```python
from build123d import *

# Parameters (mm, degrees)
SKETCH_1_W        = 29
SKETCH_1_H        = 15
SKETCH_1_R        = 1.5
SKETCH_1_R_2      = 2.5
EXTRUDE_1_DEPTH   = 3
SKETCH_1_3_R      = 4
SKETCH_1_3_R_2    = 2.5
EXTRUDE_1_2_DEPTH = 15
FILLET_1_R        = 2


with BuildPart() as part:
    # 草图1 → Extrude 1 (new body)
    # profile 1 of 2: a face of its own
    with BuildSketch(Plane.XY):
        with Locations((14.5, 7.5)):
            Rectangle(SKETCH_1_W, SKETCH_1_H)
        with Locations((9.5, 2.5)):
            Circle(SKETCH_1_R, mode=Mode.SUBTRACT)
        with Locations((9.5, 12.5)):
            Circle(SKETCH_1_R, mode=Mode.SUBTRACT)
        with Locations((26.5, 7.5)):
            Circle(SKETCH_1_R, mode=Mode.SUBTRACT)
        with Locations((2.5, 7.5)):
            Circle(SKETCH_1_R, mode=Mode.SUBTRACT)
        with Locations((14.5, 7.5)):
            Circle(SKETCH_1_R_2, mode=Mode.SUBTRACT)
    # profile 2 of 2: a face of its own
    with BuildSketch(Plane.XY):
        with Locations((14.5, 7.5)):
            Circle(SKETCH_1_R_2)
    extrude(amount=EXTRUDE_1_DEPTH)

    # 草图1<3> → Extrude 1 2 (add)
    with BuildSketch(Plane.XY):
        with Locations((14.5, 7.5)):
            Circle(SKETCH_1_3_R)
        with Locations((14.5, 7.5)):
            Circle(SKETCH_1_3_R_2, mode=Mode.SUBTRACT)
    extrude(amount=EXTRUDE_1_2_DEPTH)

    # 圆角1
    fillet_1_edges = [part.edges().sort_by_distance(p)[0] for p in [
        (0, 0, 1.5),
        (0, 15, 1.5),
        (29, 15, 1.5),
        (29, 0, 1.5),
    ]]
    fillet(fillet_1_edges, radius=FILLET_1_R)


solid = part.part
```
The listing builds one solid part. Answer for the finished solid, in the listing's coordinates (mm). A direction names the side the tool comes from. Coordinates: 2 decimals unless noted, no trailing zeros. Write each loop counter-clockwise with the first axis right and the second up, starting at its lowest first coordinate (ties: lowest second). Pieces come first, ordered by that corner, then holes.
Q1. Section B-B, the plane y = 7.5 is taken. Write down the section's boundary in (x, z), then the cut area to 3 significant figures.
Returned:
outline: (0, 0) - (1, 0) - (1, 3) - (0, 3) - close; (4, 0) - (25, 0) - (25, 3) - (18.5, 3) - (18.5, 15) - (17, 15) - (17, 3) - (12, 3) - (12, 15) - (10.5, 15) - (10.5, 3) - (4, 3) - close; (28, 0) - (29, 0) - (29, 3) - (28, 3) - close
area: 105 mm2
Q2. Find the intervals of material crossed by line 1 along X through (y, z) = (7.5, 14); line 2 along Y through (x, z) = (14.5, 9.75); line 3 along Y through (x, z) = (26.5, 1.3), in increasing order.
Returned:
line 1: x = 10.5 to 12, 17 to 18.5
line 2: y = 3.5 to 5, 10 to 11.5
line 3: y = 0 to 6, 9 to 15
Q3. Section C-C, the plane x = 9.5 is taken. Write down the section's boundary in (y, z), then the cut area to 3 significant figures.
Returned:
outline: (0, 0) - (1, 0) - (1, 3) - (0, 3) - close; (4, 0) - (11, 0) - (11, 3) - (4, 3) - close; (14, 0) - (15, 0) - (15, 3) - (14, 3) - close
area: 27.0 mm2
Q4. Which of the six approach directions +Z, -Z, +X, -X, +Y, -Y give full straight-line access (tool end or side, diameter ignored) to faces 5 (the flat face through (14, 8, 0)), 6 (the cylindrical face through (11.3, 5.1, 8.9))?
Returned:
face 5: -Z, +X, -X, +Y, -Y
face 6: +Z
Q5. Section D-D, the plane y = 12.5 is taken. Write down the section's boundary in (x, z), then the cut area to 3 significant figures.
Returned:
outline: (0, 0) - (8, 0) - (8, 3) - (0, 3) - close; (11, 0) - (29, 0) - (29, 3) - (11, 3) - close
area: 78.0 mm2
Q6. Section A-A, the plane x = 2.5 is taken. Write down the section's boundary in (y, z), then the cut area to 3 significant figures.
Returned:
outline: (0, 0) - (6, 0) - (6, 3) - (0, 3) - close; (9, 0) - (15, 0) - (15, 3) - (9, 3) - close
area: 36.0 mm2
Q7. The mould has two halves that part along X. Classify faces 1 (the cylindrical face through (12.5, 6, 8.9)), 2 (the cylindrical face through (0.57, 14.4, 1.52)), 3 (the flat face through (14, 0, 1)), 4 (the flat face through (14, 8, 3)): released by +X, released by -X, zero draft, split by the parting line, or undercut.
Returned:
face 1: undercut
face 2: released by -X
face 3: zero draft
face 4: undercut
Q8. Given P1, Ø6, axis at y = 8.5, z = 12.5, coming from the -X side; P2, Ø4, axis at x = 14.5, y = 7.5, coming from the +Z side; P3, Ø8, axis at y = 12.5, z = 13, coming from the +X side, each flat-ended and moving along its own axis, determine where each tip first touches the part or whether it passes through.
Returned:
P1: stops at x = 10.5
P2: stops at z = 3
P3: stops at x = 18.37
